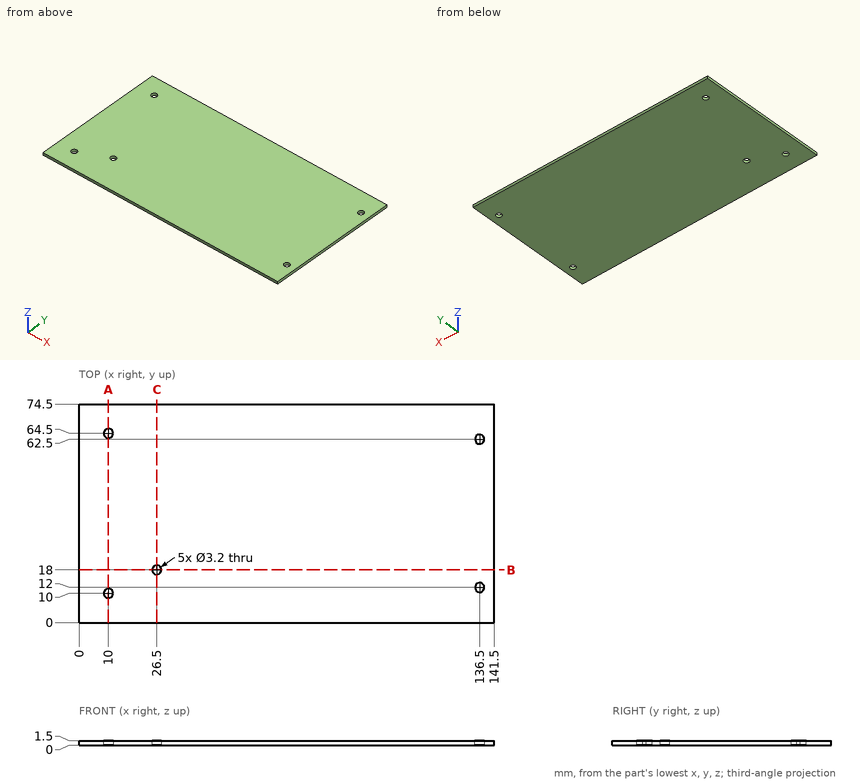
Answer from the drawing. Dimensions are ordinates in mm from the lowest x, y and z of the part. Coordinates: 2 decimals unless noted, no trailing zeros. Order: outer loops, then holes, each group sorted by start corner. A loop starts at its lowest first (then second) coordinate and runs counter-clockwise, first axis right, second up. Notation, with made-up numbers: (19, 68.5) - (26, 68.5) arc R22 ccw to (26, 107.5) - close; hole circle Ø10 at (11.5, 65.5). An arc over 180 degrees is marked (long way). Put each result on its own line as item: value. Start each with the question number.
1) Find section B-B (y = 18). Give the vertices of the cut face in (x, z).
2) Find section A-A (x = 10). Give the vertices of the cut face in (y, z), plus the area to 3 significant figures.
3) Find the intervals of material crossed by line 1 (Y direction, x = 136.5, z = 1); line 2 (Y direction, x = 10, z = 1); line 3 (X direction, y = 64.5, z = 1.2), in increasing order. Write a range as from..to.
4) Find section C-C (x = 26.5). Give the vertices of the cut face in (y, z).
Results list:
1. outline: (0, 0) - (24.9, 0) - (24.9, 1.5) - (0, 1.5) - close; (28.1, 0) - (141.5, 0) - (141.5, 1.5) - (28.1, 1.5) - close
2. outline: (0, 0) - (8.4, 0) - (8.4, 1.5) - (0, 1.5) - close; (11.6, 0) - (62.9, 0) - (62.9, 1.5) - (11.6, 1.5) - close; (66.1, 0) - (74.5, 0) - (74.5, 1.5) - (66.1, 1.5) - close
2. area: 102 mm^2
3. line 1: y = 0..10.4, 13.6..60.9, 64.1..74.5
3. line 2: y = 0..8.4, 11.6..62.9, 66.1..74.5
3. line 3: x = 0..8.4, 11.6..141.5
4. outline: (0, 0) - (16.4, 0) - (16.4, 1.5) - (0, 1.5) - close; (19.6, 0) - (74.5, 0) - (74.5, 1.5) - (19.6, 1.5) - close
